Check sheet for the drawn part. Datum: minimum x, y, z corner. Units: mm. A direction names the side the tool comes from. Round coordinates to 2 decimals unless told otherwise and drop trailing zeros. Write each loop counter-clockwise with the first axis right and the second up, starting at its lowest first coordinate (ties: lowest second). Pieces come first, ordered by that corner, then holes. Notation, with made-up numbers: (-30.5, 40.25) - (-9.5, 40.25) arc R24 ccw to (-9.5, 52.25) - close; hole circle Ø10 at (-19, 81). An arc over 180 degrees is marked (long way). Answer as a JSON object with one key per item and string values. Group by question number.
1) Set-up check for the marked faces 5, 6, 7 and 8: record each of +Z, -Z, +X, -X, +Y, -Y from which the full face is reachable in a straight line by a thin tool's end or side.
2) Thickness scan on line 1 (X direction, y = 23, z = 24); line 2 (Y direction, x = 6, z = 26.5); line 3 (Y direction, x = 50, z = 10). Record the ranges inside material, lowest first.
3) Section check D-D (y = 46.5). Enter the section's corners in (x, z).
4) Go/stop test with flat-tipped pins: pin 1 Ø12 at (x, y) = (14.5, 36) entering from +Z; pin 2 Ø10 at (x, z) = (67.5, 15.5) entering from -Y; pin 3 Ø15 at (x, z) = (104, 39.5) entering from -Y; pin 4 Ø20 at (y, z) = (46.5, 33) entering from +X. Record where each tip stops, or that it passes through.
5) Section check C-C (x = 58). Enter the section's corners in (y, z), then the cut area to 3 significant figures.
6) Section check B-B (z = 19). Enter the section's corners in (x, y), then the cut area to 3 significant figures.
7) Mould release check, pull along X, two halves, no side actions. Record for the marked faces 1, 2, 3 and 4: +X half, -X half, draft (parallel to the pull), parting line (faces both ways), or undercut.
8) Section check A-A (y = 15). Enter the section's corners in (x, z), then the cut area to 3 significant figures.
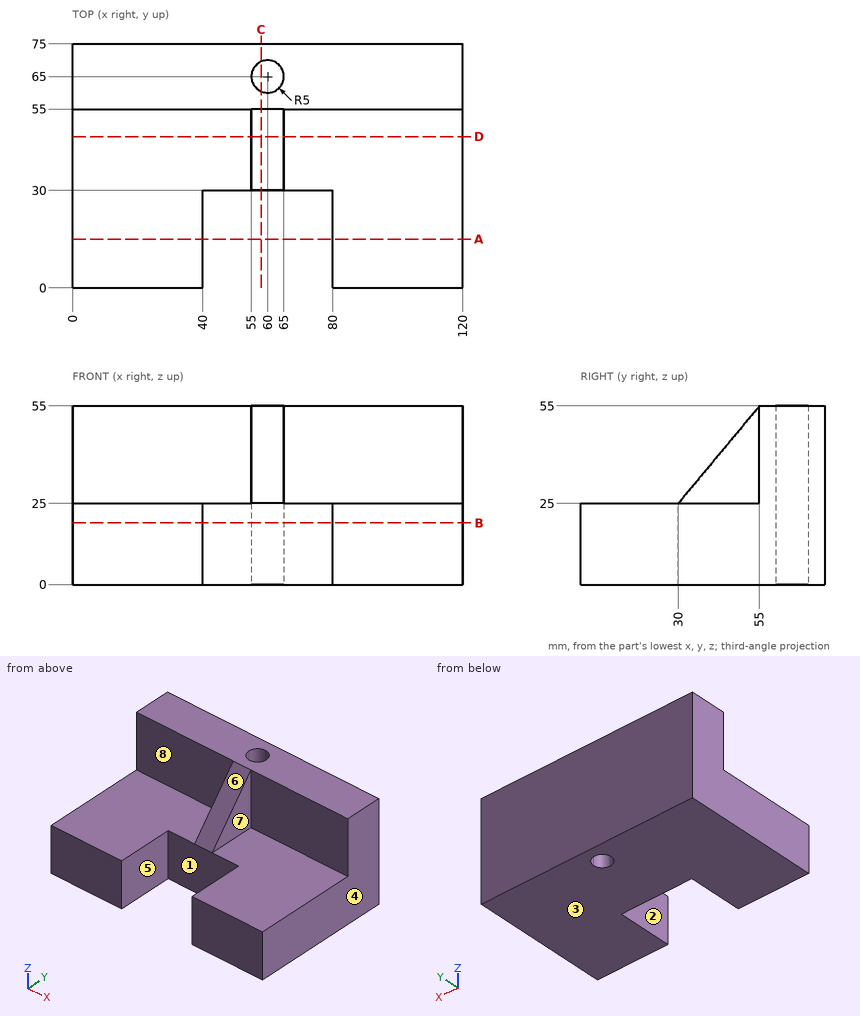
Returned:
{
 "1": {"face 5": "+Z, -Z, -Y", "face 6": "+Z, +X, -X, -Y", "face 7": "+Z, +X, -Y", "face 8": "+Z, -X, -Y"},
 "2": {"line 1": "0 to 40, 80 to 120", "line 2": "55 to 75", "line 3": "30 to 75"},
 "3": {"outline": "(0, 0) - (120, 0) - (120, 25) - (65, 25) - (65, 44.8) - (55, 44.8) - (55, 25) - (0, 25) - close"},
 "4": {"pin 1": "z = 25", "pin 2": "y = 30", "pin 3": "y = 55", "pin 4": "x = 120"},
 "5": {"outline": "(30, 0) - (60.42, 0) - (60.42, 55) - (55, 55) - (30, 25) - close; (69.58, 0) - (75, 0) - (75, 55) - (69.58, 55) - close", "area": "1,600 mm2"},
 "6": {"outline": "(0, 0) - (40, 0) - (40, 30) - (80, 30) - (80, 0) - (120, 0) - (120, 75) - (0, 75) - close; hole circle Ø10 at (60, 65)", "area": "7,720 mm2"},
 "7": {"face 1": "undercut", "face 2": "undercut", "face 3": "draft", "face 4": "+X half"},
 "8": {"outline": "(0, 0) - (40, 0) - (40, 25) - (0, 25) - close; (80, 0) - (120, 0) - (120, 25) - (80, 25) - close", "area": "2,000 mm2"}
}
